The model under review builds one solid part; all positions refer to its coordinate system, in mm. Face numbers are marked on the shaded views. Coordinates: 2 decimals unless noted, no trailing zeros. Order: outer loops, then holes, each group sorted by start corner. A loop starts at its lowest first (then second) coordinate and runs counter-clockwise, first axis right, second up.
```python
from build123d import *

# Parameters (mm, degrees)
SKETCH1_R                           = 15.875
BOSS_EXTRUDE1_DEPTH                 = 6.35
SKETCH2_R                           = 6.35
CUT_EXTRUDE1_DEPTH                  = 24.3313898
TAP_DRILL_FOR_2_56_TAP2_D           = 1.778
TAP_DRILL_FOR_2_56_TAP2_CSINK_D     = 3.048
TAP_DRILL_FOR_2_56_TAP2_CSINK_ANGLE = 100
CIRPATTERN1_COUNT                   = 2
CIRPATTERN2_COUNT                   = 2
SKETCH11_R                          = 2.286
CUT_EXTRUDE2_DEPTH                  = 24.3313898
CIRPATTERN3_COUNT                   = 2
CIRPATTERN4_COUNT                   = 3
CUT_EXTRUDE3_DEPTH                  = 24.331389963


with BuildPart() as part:
    # Sketch1 → Boss-Extrude1 (new body)
    with BuildSketch(Plane(origin=(0, 0, 0), x_dir=(1, 0, 0), z_dir=(0, 1, 0))):
        with Locations(Location((0, 0, 0), (0, 0, 270))):
            Circle(SKETCH1_R)
    extrude(amount=BOSS_EXTRUDE1_DEPTH)

    # Sketch2 → Cut-Extrude1 (cut, through all)
    with BuildSketch(Plane(origin=(0, 6.35, 0), x_dir=(1, 0, 0), z_dir=(0, 1, 0))):
        with Locations(Location((0, 0, 0), (0, 0, 270))):
            Circle(SKETCH2_R)
    extrude(amount=-CUT_EXTRUDE1_DEPTH, mode=Mode.SUBTRACT)

    # Tap Drill for #2-56 Tap2 (through all)
    with Locations(Plane(origin=(0, 6.35, 0), x_dir=(1, 0, 0), z_dir=(0, 1, 0))):
        with Locations((0, 11.1252)):
            tap_drill_for_2_56_tap2 = CounterSinkHole(TAP_DRILL_FOR_2_56_TAP2_D / 2, TAP_DRILL_FOR_2_56_TAP2_CSINK_D / 2, counter_sink_angle=TAP_DRILL_FOR_2_56_TAP2_CSINK_ANGLE)

    # CirPattern1: Tap Drill for #2-56 Tap2 ×2 about axis
    cirpattern1_axis = Axis((0, 0, 0), (0, 1, 0))
    for i in range(1, CIRPATTERN1_COUNT):
        add(tap_drill_for_2_56_tap2.rotate(cirpattern1_axis, i * 360 / CIRPATTERN1_COUNT), mode=Mode.SUBTRACT)

    # Sketch10 → Tap Drill for #2-56 Tap1 (revolve, cut)
    with BuildSketch(Plane(origin=(11.1252, 6.35, 0), x_dir=(0, 0, 1), z_dir=(1, 0, 0))):
        Polygon((0, 0), (0, 4.34416509), (0.889, 3.81), (0.889, 0.532828266), (1.524, 0), align=None)
    tap_drill_for_2_56_tap1 = revolve(axis=Axis((11.1252, 12.7, 0), (0, -1, 0)), mode=Mode.SUBTRACT)

    # CirPattern2: Tap Drill for #2-56 Tap1 ×2 about axis
    cirpattern2_axis = Axis((0, 0, 0), (0, 1, 0))
    for i in range(1, CIRPATTERN2_COUNT):
        add(tap_drill_for_2_56_tap1.rotate(cirpattern2_axis, i * 360 / CIRPATTERN2_COUNT), mode=Mode.SUBTRACT)

    # Sketch11 → Cut-Extrude2 (cut, through all)
    with BuildSketch(Plane(origin=(0, 6.35, 0), x_dir=(1, 0, 0), z_dir=(0, 1, 0))):
        with Locations(Location((-7.360856908, 8.324988999, 0), (0, 0, 270))):
            Circle(SKETCH11_R)
    cut_extrude2 = extrude(amount=-CUT_EXTRUDE2_DEPTH, mode=Mode.SUBTRACT)

    # CirPattern3: Cut-Extrude2 ×2 about axis
    cirpattern3_axis = Axis((0, 0, 0), (0, 1, 0))
    for i in range(1, CIRPATTERN3_COUNT):
        add(cut_extrude2.rotate(cirpattern3_axis, i * 360 / CIRPATTERN3_COUNT), mode=Mode.SUBTRACT)

    # Sketch16 → Tap Drill for #2-56 Tap3 (revolve, cut)
    with BuildSketch(Plane(origin=(12.093135875, 3.244987275, -10.284536436), x_dir=(-0.6478448148472237, 0, -0.7617723386127685), z_dir=(0, 1, 0))):
        Polygon((0, 0), (0, 7.095959572), (0.889, 6.35), (0.889, 0), align=None)
    tap_drill_for_2_56_tap3 = revolve(axis=Axis((16.930390226, 3.244987275, -14.39835101), (-0.7617723386127686, 0, 0.6478448148472237)), mode=Mode.SUBTRACT)

    # CirPattern4: Tap Drill for #2-56 Tap3 ×3 about axis
    cirpattern4_axis = Axis((0, 6.35, 0), (0, -1, 0))
    for i in range(1, CIRPATTERN4_COUNT):
        add(tap_drill_for_2_56_tap3.rotate(cirpattern4_axis, i * 360 / CIRPATTERN4_COUNT), mode=Mode.SUBTRACT)

    # Sketch17 → Cut-Extrude3 (cut, through all)
    with BuildSketch(Plane(origin=(0, 6.35, 0), x_dir=(1, 0, 0), z_dir=(0, 1, 0))):
        with BuildLine():
            Line((-4.96914615, -6.489934512), (-6.955810814, -4.646503161))
            ThreePointArc((-6.955810814, -4.646503161), (-6.979764598, -4.005972756), (-6.339234193, -3.982018972))
            Line((-6.339234193, -3.982018972), (-4.352569529, -5.825450323))
            ThreePointArc((-4.352569529, -5.825450323), (-4.328615745, -6.465980728), (-4.96914615, -6.489934512))
        make_face()
    extrude(amount=-CUT_EXTRUDE3_DEPTH, mode=Mode.SUBTRACT)


solid = part.part
```
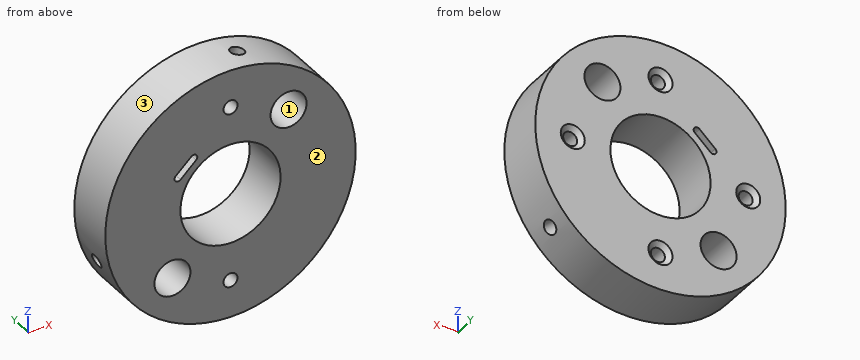
(1) We need section D-D, the plane x = 13.5. Write out the cut boundary in (y, z).
A:
outline: (0, -8.35) - (6.35, -8.35) - (6.35, 8.35) - (0, 8.35) - close
(2) Wall thickness on probe 1 along X at (y, z) = (4.1, 0) (3 decimals); probe 2 along X at (y, z) = (3, 9); probe 3 along X at (y, z) = (3.5, 3): over which ranges is each line inside the solid? List them lowest first.
A:
probe 1: x = -15.875 to -12.014, -10.236 to -6.35, 6.35 to 10.236, 12.014 to 15.875
probe 2: x = -13.08 to 1.35, 2.15 to 5.18, 9.54 to 13.08
probe 3: x = -15.59 to -5.6, 5.6 to 15.59
(3) We need section A-A, the plane x = 0. Write out the cut boundary in (y, z) (3 decimals), and give its area (3 significant figures).
A:
outline: (0, -15.875) - (6.35, -15.875) - (6.35, -12.649) - (5.817, -12.014) - (0, -12.014) - close; (0, -10.236) - (5.817, -10.236) - (6.35, -9.601) - (6.35, -6.35) - (0, -6.35) - close; (0, 6.35) - (6.35, 6.35) - (6.35, 9.601) - (5.817, 10.236) - (0, 10.236) - close; (0, 12.014) - (5.817, 12.014) - (6.35, 12.649) - (6.35, 15.875) - (0, 15.875) - close
area: 97.7 mm2
(4) We need section B-B, the plane y = 4.75. Count the separate pieces of the cut face and the enclosed holes in it, and give its area (3 significant figures).
A:
separate pieces: 1
enclosed holes: 8
area: 619 mm2
(5) For pin 1 Ø1.5 at (x, y) = (-8, 5.5) entering from -Z; pin 2 Ø1.6 at (x, z) = (0, 11.13) entering from -Y; pin 3 Ø3 at (x, y) = (-10.5, 5.5) entering from +Z, all flat-tipped, find the tip position at first contact; note any pin that passes through.
A:
pin 1: stops at z = -14.12
pin 2: passes through
pin 3: stops at z = 13.08
(6) Draft analysis for pull direction X (two halves, no side actions). For the marked faces 1, 2 and 3, state which applies: released by +X, released by -X, zero draft, split by the parting line, or undercut.
A:
face 1: undercut
face 2: zero draft
face 3: split by the parting line
